```python
from build123d import *

# Parameters (mm, degrees)
SKETCH_1_R          = 7
EXTRUDE_1_DEPTH     = 1.5
SKETCH_2_R          = 6
EXTRUDE_2_DEPTH     = 2.5
SKETCH_3_R          = 3.9
CUT_EXTRUDE_1_DEPTH = 11.677078252


with BuildPart() as part:
    # 草图1 → 凸台-拉伸1 (new body)
    with BuildSketch(Plane(origin=(0, 0, 0), x_dir=(1, 0, 0), z_dir=(0, 1, 0))):
        with Locations(Location((0, 0, 0), (0, 0, 270))):
            Circle(SKETCH_1_R)
    extrude(amount=EXTRUDE_1_DEPTH)

    # 草图2 → 凸台-拉伸2 (add)
    with BuildSketch(Plane(origin=(0, 1.5, 0), x_dir=(1, 0, 0), z_dir=(0, 1, 0))):
        with Locations(Location((0, 0, 0), (0, 0, 270))):
            Circle(SKETCH_2_R)
    extrude(amount=EXTRUDE_2_DEPTH)

    # 草图3 → 切除-拉伸1 (cut, through all)
    with BuildSketch(Plane(origin=(0, 4, 0), x_dir=(1, 0, 0), z_dir=(0, 1, 0))):
        with Locations(Location((0, 0, 0), (0, 0, 270))):
            Circle(SKETCH_3_R)
    extrude(amount=-CUT_EXTRUDE_1_DEPTH, mode=Mode.SUBTRACT)


with BuildPart() as part_1:
    # Move Body 1: moved
    add(part.part.moved(Location((-171.120476201, -93.573160839, 270.177536174))))


solid = part_1.part
```
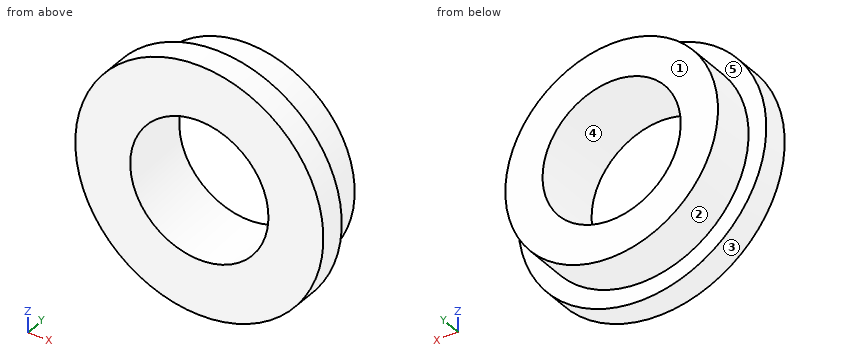
Can you work these out from the model? Positions are in its coordinate system, mm. Face numbers are marked on the shaded views. A direction names the side the tool comes from. Round coordinates to 2 decimals unless told otherwise and drop trailing zeros. Loops run counter-clockwise (first coordinate to the right, second up) from the corner with the lowest first, then second, coordinate; pieces in that order, holes last. Notation, with made-up numbers: M -25.5,-16 L 17.5,-16 A23 ccw 17.5,11 Z; hole C 13.5,65.5 d11. An arc over 180 degrees is marked long. Answer as a JSON object with one key per item and string values. Group by question number.
Q1. Please list where these lines run through material, in increasing order: L1, parallel to Z at x = -173, y = -90; L2, parallel to Y at x = -170.25, z = 276.25; L3, parallel to X at y = -93.3, z = 269.5.
Q2. Imagine slicing it at D-D, the plane y = -91.85. Please give me the cut outline in (x, z).
Q3. Imagine slicing it at C-C, the plane z = 264.5. Please give me the cut outline in (x, y), then the cut area to 3 significant figures.
Q4. On a 3-axis mill with a long thin cutter (end or side, diameter ignored), from which of +Z, -Z, +X, -X, +Y, -Y can I reach the whole of each face in a straight line? I mean the marked faces 1 and 2. Say none if no direction works.
Q5. Will these pins go through, and if not, where does the flat tip stop? pin 1 (1.5 mm diameter, centred on x = -166.5, y = -92, fed in from -Z); pin 2 (5 mm diameter, centred on x = -171, z = 270.5, fed in from -Y); pin 3 (1.5 mm diameter, centred on x = -167, y = -92, fed in from +Z).
Q6. Imagine slicing it at A-A, the plane x = -170.5. Please give me the cut outline in (y, z), then the cut area to 3 significant figures.
Q7. We'd pull the mould along Z, two halves only. Please class the marked faces 3, 4 and 5: +Z half, -Z half, draft (parallel to the pull), parting line (faces both ways), or undercut.
Q8. Imagine slicing it at B-B, the plane z = 273.25. Please give me the cut outline in (x, y), then the cut area to 3 significant figures.
Findings:
{
 "1": {"L1": "z = 264.48 to 266.76, 273.59 to 275.88", "L2": "y = -93.57 to -92.07", "L3": "x = -178.09 to -174.96, -167.28 to -164.15"},
 "2": {"outline": "C -171.12,270.18 d12; hole C -171.12,270.18 d7.8"},
 "3": {"outline": "M -175.22,-93.57 L -167.03,-93.57 L -167.03,-92.07 L -169.18,-92.07 L -169.18,-89.57 L -173.06,-89.57 L -173.06,-92.07 L -175.22,-92.07 Z", "area": "22.0 mm2"},
 "4": {"face 1": "+Z, -Z, +X, -X, +Y", "face 2": "+Y"},
 "5": {"pin 1": "stops at z = 264.35", "pin 2": "passes through", "pin 3": "stops at z = 276.31"},
 "6": {"outline": "M -93.57,263.21 L -92.07,263.21 L -92.07,264.21 L -89.57,264.21 L -89.57,266.33 L -93.57,266.33 Z; M -93.57,274.03 L -89.57,274.03 L -89.57,276.15 L -92.07,276.15 L -92.07,277.15 L -93.57,277.15 Z", "area": "20.0 mm2"},
 "7": {"face 3": "parting line", "face 4": "undercut", "face 5": "draft"},
 "8": {"outline": "M -177.41,-93.57 L -173.52,-93.57 L -173.52,-89.57 L -176.27,-89.57 L -176.27,-92.07 L -177.41,-92.07 Z; M -168.72,-93.57 L -164.83,-93.57 L -164.83,-92.07 L -165.97,-92.07 L -165.97,-89.57 L -168.72,-89.57 Z", "area": "25.4 mm2"}
}
